Check sheet for the modelled part. Datum: model origin and axes. Units: mm. A direction names the side the tool comes from. Give positions to 0.01 mm unless a question says otherwise; leave off trailing zeros. Order: outer loops, then holes, each group sorted by start corner. A loop starts at its lowest first (then second) coordinate and runs counter-clockwise, first axis right, second up.
Autodesk Inventor part; units mm, degrees
ref_plane "YZ Plane" through (0, 0, 0) normal (1, 0, 0) x (0, 1, 0)
ref_plane "XZ Plane" through (0, 0, 0) normal (0, 1, 0) x (-1, 0, 0)
ref_plane "XY Plane" through (0, 0, 0) normal (0, 0, 1) x (1, 0, 0)
sketch "Sketch1" plane through (0, 0, 0) normal (0, 1, 0) x (-1, 0, 0)
  line L0 (64, -147.5) -> (-64, -147.5)
  line L1 (-64, -147.5) -> (-64, 147.5)
  line L2 (-64, 147.5) -> (64, 147.5)
  line L3 (64, 147.5) -> (64, -147.5)
  line L4 (64, -147.5) -> (-64, 147.5) construction
  line L5 (-64, -147.5) -> (64, 147.5) construction
  point P0 (0, 0)
  dimension "d0" = 128
  dimension "d1" = 295
extrude "Extrusion1" add sketch "Sketch1" along normal blind 3
sketch "Sketch2" plane through (0, 0, 0) normal (0, -1, 0) x (1, 0, 0)
  line L0 (-57.5, 25) -> (-57.5, -25) construction
  line L1 (-65, 25) -> (-65, -25)
  line L2 (-50, -25) -> (-50, 25)
  arc A0 (-50, 25) -> (-65, 25) centre (-57.5, 25) ccw
  arc A1 (-65, -25) -> (-50, -25) centre (-57.5, -25) ccw
  line L3 (-57.5, 0) -> (-7.5, 0) construction
  point P0 (0, 0)
  dimension "d4" = 25
  dimension "d5" = 90
  dimension "d6" = 15
  dimension "d7" = 50
extrude "Extrusion2" cut sketch "Sketch2" against normal blind 3
sketch "Sketch3" plane through (0, 0, 0) normal (0, -1, 0) x (1, 0, 0)
  line L0 (30, -30) -> (-30, -30)
  line L1 (-30, -30) -> (-30, 30)
  line L2 (-30, 30) -> (30, 30)
  line L3 (30, 30) -> (30, -30)
  line L4 (30, -30) -> (-30, 30) construction
  line L5 (-30, -30) -> (30, 30) construction
  circle A0 centre (-25, -25) radius 2.2
  circle A1 centre (-25, 25) radius 2.2
  circle A2 centre (25, 25) radius 2.2
  circle A3 centre (25, -25) radius 2.2
  circle A4 centre (0, 0) radius 27.5
  dimension "d10" = 60
  dimension "d11" = 60
  dimension "d12" = 4.4
  dimension "d13" = 5
  dimension "d14" = 4.4
  dimension "d15" = 4.4
  dimension "d16" = 4.4
  dimension "d17" = 5
  dimension "d18" = 5
  dimension "d19" = 5
  dimension "d20" = 55
extrude "Extrusion3" cut sketch "Sketch3" against normal blind 3 contours A0 | A1 | A2 | A3 | A4
sketch "Sketch5" plane through (0, 0, 0) normal (0, -1, 0) x (1, 0, 0)
  circle A0 centre (14, -97.5) radius 1.375
  circle A1 centre (-44, -97.5) radius 1.375
  circle A2 centre (-44, -48.5) radius 1.375
  circle A3 centre (14, -48.5) radius 1.375
  line L0 (-64, 147.5) -> (-64, -147.5)
  line L1 (-64, -147.5) -> (64, -147.5)
  point P0 (0, 0)
  dimension "d23" = 2.75
  dimension "d24" = 2.75
  dimension "d25" = 2.75
  dimension "d26" = 2.75
  dimension "d27" = 58
  dimension "d28" = 58
  dimension "d29" = 49
  dimension "d30" = 20
  dimension "d31" = 50
  dimension "d32" = 50
  dimension "d33" = 20
  dimension "d36" = 49
extrude "Extrusion4" cut sketch "Sketch5" against normal blind 3
sketch "Sketch6" plane through (0, 0, 0) normal (0, -1, 0) x (1, 0, 0)
  line L0 (-40, -89.5) -> (-6, -89.5)
  line L1 (-6, -69.5) -> (-6, -55.5)
  line L2 (-7, -54.5) -> (-40, -54.5)
  line L3 (-41, -55.5) -> (-41, -88.5)
  circle A0 centre (-44, -97.5) radius 1.375
  circle A1 centre (-44, -48.5) radius 1.375
  line L4 (-6, -89.5) -> (8, -89.5)
  line L5 (9, -88.5) -> (9, -75.5)
  line L6 (8, -74.5) -> (-1, -74.5)
  line L7 (-6, -74.5) -> (-6, -89.5)
  arc A2 (-6, -69.5) -> (-1, -74.5) centre (-1, -69.5) ccw
  arc A3 (9, -75.5) -> (8, -74.5) centre (8, -75.5) ccw
  arc A4 (8, -89.5) -> (9, -88.5) centre (8, -88.5) ccw
  arc A5 (-41, -88.5) -> (-40, -89.5) centre (-40, -88.5) ccw
  arc A6 (-40, -54.5) -> (-41, -55.5) centre (-40, -55.5) ccw
  arc A7 (-6, -55.5) -> (-7, -54.5) centre (-7, -55.5) ccw
  point P0 (0, 0)
  point P1 (9, -74.5)
  point P2 (9, -89.5)
  dimension "d39" = 3
  dimension "d43" = 6
  dimension "d58" = 15
  dimension "d59" = 15
  dimension "d60" = 5
  dimension "d61" = 1
extrude "Extrusion5" cut sketch "Sketch6" against normal blind 3 contours A5 L3 A6 L2 A7 L1 A2 L6 A3 L5 A4 L4 L0
sketch "Sketch8" plane through (0, 0, 0) normal (0, -1, 0) x (1, 0, 0)
  circle A0 centre (-14, 97.5) radius 12.5
  line L0 (64, 147.5) -> (-64, 147.5)
  line L1 (-64, 147.5) -> (-64, 28.7417)
  circle A1 centre (26, 97.5) radius 8.5
  point P0 (0, 0)
  dimension "d44" = 25
  dimension "d45" = 50
  dimension "d46" = 50
  dimension "d49" = 17
  dimension "d50" = 50
  dimension "d51" = 40
extrude "Extrusion6" cut sketch "Sketch8" against normal blind 3
fillet "Fillet1" radius 2 2 edges at (-64, 1.5, 28.7417) (-64, 1.5, -28.7417)
sketch "Sketch9" plane through (0, 0, 0) normal (0, -1, 0) x (1, 0, 0)
  line L0 (-5, 51.815) -> (5, 51.815)
  line L1 (5, 51.815) -> (5, 41.815)
  line L2 (5, 41.815) -> (-5, 41.815)
  line L3 (-5, 41.815) -> (-5, 51.815)
  line L4 (-5, 51.815) -> (5, 41.815) construction
  line L5 (5, 51.815) -> (-5, 41.815) construction
  point P0 (0, 0)
  point P1 (0, 46.815)
  dimension "d53" = 10
  dimension "d54" = 10
  dimension "d55" = 0
extrude "Extrusion7" cut sketch "Sketch9" against normal blind 10
fillet "Fillet2" radius 10 2 edges at (-64, 1.5, 147.5) (-64, 1.5, -147.5)
properties part number "binnenplaat"
(1) Cross-section at A-A on z = -82.5. Enter the section's corners in (x, y).
Response values:
outline: (-64, 0) - (-41, 0) - (-41, 3) - (-64, 3) - close; (9, 0) - (64, 0) - (64, 3) - (9, 3) - close
(2) Cross-section at C-C on z = 7.5. Enter the section's corners in (x, y).
Response values:
outline: (-50, 0) - (-26.46, 0) - (-26.46, 3) - (-50, 3) - close; (26.46, 0) - (64, 0) - (64, 3) - (26.46, 3) - close
(3) Gauge pin test, flat ends, axial feed: pin 1 Ø1.6 at (x, z) = (14, -48.5) entering from -Y; pin 2 Ø1.5 at (y, z) = (2, 12.5) entering from -X. Record the tip position at first contact, or that the pin passes through.
Response values:
pin 1: passes through
pin 2: stops at x = -50
(4) Material ranges on L1, parallel to Z at x = 14, y = 1.85 (3 decimals); L2, parallel to Z at x = -11, y = 2.3; L3, parallel to Z at x = 5.5, y = 2.2, recorded low to high.
Response values:
L1: z = -147.5 to -98.875, -96.125 to -49.875, -47.125 to -23.67, 23.67 to 147.5
L2: z = -147.5 to -89.5, -54.5 to -25.2, 25.2 to 85.37, 109.63 to 147.5
L3: z = -147.5 to -89.5, -74.5 to -26.94, 26.94 to 147.5
(5) Cross-section at B-B on y = 2.55. Count the separate pieces of the cut face and the enclosed holes in it, then the cut area to 3 significant figures.
Response values:
separate pieces: 1
enclosed holes: 13
area: 32,100 mm2
(6) Release check for a two-part mould opening along Z. For faces 1 (the face through (29, 0, 2)), 2 (the face through (-4.57, 1.48, -73)), 3 (the face through (-60.99, 1.52, -144.65)), 4 (the face through (-53.56, 1.48, 31.38)) record: released by +Z, released by -Z, zero draft, split by the parting line, or undercut.
Response values:
face 1: zero draft
face 2: undercut
face 3: released by -Z
face 4: undercut
(7) Set-up check for faces 5 (the face through (-53.746, 1.479, -31.493)), 6 (the face through (29, 3, 2)): record each of +Z, -Z, +X, -X, +Y, -Y from which the full face is reachable in a straight line by a thin tool's end or side.
Response values:
face 5: +Y, -Y
face 6: +Z, -Z, +X, -X, +Y
